Autodesk Inventor part; units mm, degrees
ref_plane "YZ Plane" through (0, 0, 0) normal (1, 0, 0) x (0, 1, 0)
ref_plane "XZ Plane" through (0, 0, 0) normal (0, 1, 0) x (-1, 0, 0)
ref_plane "XY Plane" through (0, 0, 0) normal (0, 0, 1) x (1, 0, 0)
sketch "Sketch1" plane through (0, 0, 0) normal (0, 1, 0) x (-1, 0, 0)
  line L0 (-95.7688, 101.9192) -> (4.2312, 101.9192)
  line L1 (4.2312, 101.9192) -> (4.2312, 1.9192)
  line L2 (4.2312, 1.9192) -> (-95.7688, 1.9192)
  line L3 (-95.7688, 1.9192) -> (-95.7688, 101.9192)
  line L4 (-95.7688, 1.9192) -> (4.2312, 1.9192)
  line L5 (4.2312, 1.9192) -> (4.2312, 6.9192)
  line L6 (4.2312, 6.9192) -> (-95.7688, 6.9192)
  line L7 (-95.7688, 6.9192) -> (-95.7688, 1.9192)
  line L8 (4.2312, 1.9192) -> (-15.7688, 1.9192)
  line L9 (-15.7688, 1.9192) -> (-15.7688, 32.9192)
  line L10 (-15.7688, 32.9192) -> (4.2312, 32.9192)
  line L11 (4.2312, 32.9192) -> (4.2312, 1.9192)
  line L12 (-95.7688, 1.9192) -> (-75.7688, 1.9192)
  line L13 (-75.7688, 1.9192) -> (-75.7688, 32.9192)
  line L14 (-75.7688, 32.9192) -> (-95.7688, 32.9192)
  line L15 (-95.7688, 32.9192) -> (-95.7688, 1.9192)
  point P0 (0, 0)
  dimension "d0" = 100
  dimension "d1" = 100
  dimension "d2" = 5
  dimension "d3" = 20
  dimension "d4" = 31
  dimension "d5" = 20
extrude "Extrusion1" add sketch "Sketch1" along normal blind 2 contours L0 L1 L10 L9 L6 L13 L14 L3 | L6 L9 L2 L13
sketch "Sketch2" plane through (0, 2, 0) normal (0, 1, 0) x (1, 0, 0)
  line L0 (-4.2312, -82.6348) -> (-4.2312, -11.6268)
  line L1 (95.7688, -11.6268) -> (95.7688, -82.6348)
  line L2 (75.7688, -32.9192) -> (75.7688, -1.9192)
  line L3 (15.7688, -1.9192) -> (15.7688, -32.9192)
  line L4 (75.7688, -1.9192) -> (15.7688, -1.9192)
  line L5 (15.7688, -1.9192) -> (15.7688, -6.9192)
  line L6 (15.7688, -6.9192) -> (75.7688, -6.9192)
  line L7 (75.7688, -6.9192) -> (75.7688, -1.9192)
  line L8 (95.7688, -82.6348) -> (-4.2312, -82.6348)
  line L9 (95.7688, -11.6268) -> (-4.2312, -11.6268)
  point P0 (0, 0)
  dimension "d8" = 5
extrude "Extrusion2" cut sketch "Sketch2" against normal blind 2 contours L3 L4 L2 L6
sketch "Szkic3" plane through (0, 2, 0) normal (0, 1, 0) x (1, 0, 0)
  circle A0 centre (66.0188, -29.6192) radius 1.75
  circle A1 centre (25.5188, -29.6192) radius 1.75
  point P0 (0, 0)
extrude "Wyciągnięcie proste3" cut sketch "Szkic3" against normal through all
sketch "Szkic4" plane through (0, 0, 0) normal (0, -1, 0) x (1, 0, 0)
  circle A0 centre (25.5188, 29.6192) radius 1.75
  circle A1 centre (66.0188, 29.6192) radius 1.75
  line L0 (15.7688, 6.9192) -> (75.7688, 6.9192)
  line L1 (75.7688, 32.9192) -> (75.7688, 6.9192)
  line L2 (95.7688, 32.9192) -> (75.7688, 32.9192)
  line L3 (95.7688, 101.9192) -> (95.7688, 32.9192)
  line L4 (-4.2312, 101.9192) -> (95.7688, 101.9192)
  line L5 (-4.2312, 32.9192) -> (-4.2312, 101.9192)
  line L6 (15.7688, 32.9192) -> (-4.2312, 32.9192)
  line L7 (15.7688, 6.9192) -> (15.7688, 32.9192)
  point P0 (0, 0)
extrude "Wyciągnięcie proste4" add sketch "Szkic4" against normal up to surface (2 mm away) contours A0 | A1
sketch "Szkic5" plane through (0, 2, 0) normal (0, 1, 0) x (1, 0, 0)
  circle A0 centre (22.8938, -32.6829) radius 1.5
  circle A1 centre (68.6438, -32.6829) radius 1.5
  point P0 (0, 0)
extrude "Wyciągnięcie proste5" cut sketch "Szkic5" against normal through all
sketch "Szkic6" plane through (-4.2312, 0, 101.9192) normal (0, 0, 1) x (1, 0, 0)
  line L0 (0, 0) -> (100, 0)
  line L1 (100, 0) -> (100, 2)
  line L2 (0, 2) -> (100, 2)
  line L3 (0, 0) -> (0, 2)
  point P0 (4.2312, 0)
extrude "Wyciągnięcie proste6" cut sketch "Szkic6" against normal blind 2.5
sketch "Szkic7" plane through (0, 0, 0) normal (0, -1, 0) x (1, 0, 0)
  circle A0 centre (1.7688, 72.4703) radius 1.5
  circle A1 centre (8.7688, 39.9192) radius 1.5
  point P0 (0, 0)
extrude "Wyciągnięcie proste7" cut sketch "Szkic7" against normal through all
sketch "Szkic8" plane through (0, 0, 0) normal (0, -1, 0) x (1, 0, 0)
  circle A0 centre (8.7688, 39.9192) radius 1.5
  circle A1 centre (1.7688, 72.4703) radius 1.5
  line L0 (95.7688, 99.4192) -> (-4.2312, 99.4192)
  line L1 (-4.2312, 32.9192) -> (-4.2312, 99.4192)
  line L2 (15.7688, 32.9192) -> (-4.2312, 32.9192)
  line L3 (15.7688, 6.9192) -> (15.7688, 32.9192)
  line L4 (15.7688, 6.9192) -> (75.7688, 6.9192)
  line L5 (75.7688, 32.9192) -> (75.7688, 6.9192)
  line L6 (95.7688, 32.9192) -> (75.7688, 32.9192)
  line L7 (95.7688, 99.4192) -> (95.7688, 32.9192)
  circle A2 centre (22.8938, 32.6829) radius 1.5
  circle A3 centre (68.6438, 32.6829) radius 1.5
  line L8 (-4.2312, 39.9192) -> (21.3688, 39.9192)
  circle A4 centre (21.3688, 39.9192) radius 2.1391
  line L9 (-4.2312, 32.9192) -> (-4.2312, 60.9192)
  line L10 (-4.2312, 32.9192) -> (-4.2312, 99.4192)
  point P0 (0, 0)
  dimension "d21" = 25.6
  dimension "d22" = 28
sketch "Szkic9" plane through (0, 0, 0) normal (0, -1, 0) x (1, 0, 0)
  circle A0 centre (25.5188, 29.6192) radius 1.75
  circle A1 centre (66.0188, 29.6192) radius 1.75
  point P0 (0, 0)
extrude "Wyciągnięcie proste8" cut sketch "Szkic9" against normal through all
extrude "Wyciągnięcie proste9" add sketch "Szkic8" against normal up to surface (2 mm away) contours A2 | A3
sketch "Szkic10" plane through (0, 0, 0) normal (0, -1, 0) x (1, 0, 0)
  circle A0 centre (45.7688, 11.3479) radius 1.5
  point P0 (0, 0)
extrude "Wyciągnięcie proste10" cut sketch "Szkic10" against normal through all
properties part number "minisumopodsr" material "Aluminum 6061"
The model under review builds one solid part; all positions refer to its coordinate system, in mm. Round coordinates to 2 decimals unless told otherwise and drop trailing zeros. Write each loop counter-clockwise with the first axis right and the second up, starting at its lowest first coordinate (ties: lowest second). Pieces come first, ordered by that corner, then holes.
(1) We need section B-B on y = 0.95. Give the boundary of the cut face in (x, z).
(2) Mouldability with a two-part tool opening along X and no side actions: class faces 1 (the flat face through (46, 0, 54)), 2 (the cylindrical face through (65.64, 0.99, 27.91)), 3 (the cylindrical face through (8.444, 0.986, 38.455)) as +X half, -X half, draft (parallel to the pull), parting line (faces both ways), or undercut.
(3) Wall thickness on L1, parallel to Z at x = 78.5, y = 0.5; L2, parallel to Z at x = 27, y = 1.8; L3, parallel to Z at x = 2.5, y = 1.6: over which ranges is each line inside the solid? List them lowest first.
(4) We need section D-D on x = 77. Give the boundary of the cut face in (y, z).
(5) Insertion check: pin 1 (1 mm diameter, centred on x = 13.5, y = 1, fed in from -Z); pin 2 (1 mm diameter, centred on y = 1.5, z = 23.5, fed in from -X). Each pin has a flat end and moves straight along its axis. Give the tip position at first contact, or say it passes through.
(6) We need section A-A on x = 2. Give the boundary of the cut face in (y, z), and give its area (3 significant figures).
(7) We need section C-C on z = 18.5. Give the boundary of the cut face in (x, y).
Findings below:
1. outline: (-4.23, 32.92) - (15.77, 32.92) - (15.77, 6.92) - (75.77, 6.92) - (75.77, 32.92) - (95.77, 32.92) - (95.77, 99.42) - (-4.23, 99.42) - close; hole circle Ø3 at (1.77, 72.47); hole circle Ø3 at (8.77, 39.92); hole circle Ø3.5 at (25.52, 29.62); hole circle Ø3 at (45.77, 11.35); hole circle Ø3.5 at (66.02, 29.62)
2. face 1: draft
2. face 2: undercut
2. face 3: undercut
3. L1: z = 32.92 to 99.42
3. L2: z = 6.92 to 28.69, 30.55 to 99.42
3. L3: z = 32.92 to 71.16, 73.78 to 99.42
4. outline: (0, 32.92) - (2, 32.92) - (2, 99.42) - (0, 99.42) - close
5. pin 1: stops at z = 32.92
5. pin 2: stops at x = 15.77
6. outline: (0, 32.92) - (2, 32.92) - (2, 70.99) - (0, 70.99) - close; (0, 73.95) - (2, 73.95) - (2, 99.42) - (0, 99.42) - close
6. area: 127 mm2
7. outline: (15.77, 0) - (75.77, 0) - (75.77, 2) - (15.77, 2) - close
